Check sheet for the modelled part. Datum: model origin and axes. Units: mm. Face numbers are marked on the shaded views. A direction names the side the tool comes from. Coordinates: 2 decimals unless noted, no trailing zeros. Loops run counter-clockwise (first coordinate to the right, second up) from the corner with the lowest first, then second, coordinate; pieces in that order, holes last. Notation, with made-up numbers: M 26,-38 L 55,-38 A29 cw 55,-3 Z; hole C -13,-21.75 d2. An arc over 180 degrees is marked long. Return JSON: item names as keys, results as strings.
from build123d import *

# Parameters (mm, degrees)
SKETCH2_W                   = 191
SKETCH2_H                   = 130
BOSS_EXTRUDE1_DEPTH         = 35
SKETCH10_W                  = 35
SKETCH10_H                  = 130
BOSS_EXTRUDE2_DEPTH         = 101
TAP_DRILL_FOR_M4_TAP2_D     = 3.3
TAP_DRILL_FOR_M4_TAP2_DEPTH = 6
TAP_DRILL_FOR_M4_TAP2_TIP   = 0.991420021
TAP_DRILL_FOR_M4_TAP3_D     = 3.3
TAP_DRILL_FOR_M4_TAP3_DEPTH = 6
TAP_DRILL_FOR_M4_TAP3_TIP   = 0.991420021
CUT_EXTRUDE1_DEPTH          = 205.770603359
F_8_0MM_DOWEL_HOLE1_D       = 8
CUT_EXTRUDE3_DEPTH          = 30
F_8_0MM_DOWEL_HOLE2_D       = 8
F_8_0MM_DOWEL_HOLE2_DEPTH   = 10
F_8_0MM_DOWEL_HOLE2_TIP     = 2.403442476
F_12_0MM_DOWEL_HOLE1_D      = 12
F_12_0MM_DOWEL_HOLE1_DEPTH  = 10
F_12_0MM_DOWEL_HOLE1_TIP    = 3.605163714


with BuildPart() as part:
    # Sketch2 → Boss-Extrude1 (new body)
    with BuildSketch(Plane(origin=(0, 0, 0), x_dir=(0, 0, -1), z_dir=(1, 0, 0))):
        with Locations((95.5, 0)):
            Rectangle(SKETCH2_W, SKETCH2_H)
    extrude(amount=BOSS_EXTRUDE1_DEPTH)

    # Sketch10 → Boss-Extrude2 (add)
    with BuildSketch(Plane.XY):
        with Locations((17.5, 0)):
            Rectangle(SKETCH10_W, SKETCH10_H)
    extrude(amount=BOSS_EXTRUDE2_DEPTH)

    # Tap Drill for M4 Tap2
    with Locations(Plane(origin=(0, 0, -191), x_dir=(-1, 0, 0), z_dir=(0, 0, -1))):
        with Locations((-40, 35), (-10, 35), (-10, -35), (-40, -35)):
            Hole(TAP_DRILL_FOR_M4_TAP2_D / 2, depth=TAP_DRILL_FOR_M4_TAP2_DEPTH)
            with Locations((0, 0, -(TAP_DRILL_FOR_M4_TAP2_DEPTH + TAP_DRILL_FOR_M4_TAP2_TIP / 2))):  # 118° drill point
                Cone(0, TAP_DRILL_FOR_M4_TAP2_D / 2, TAP_DRILL_FOR_M4_TAP2_TIP, mode=Mode.SUBTRACT)

    # Tap Drill for M4 Tap3
    with Locations(Plane.XY.offset(101)):
        with Locations((10, 35), (40, 35), (40, -35), (10, -35)):
            Hole(TAP_DRILL_FOR_M4_TAP3_D / 2, depth=TAP_DRILL_FOR_M4_TAP3_DEPTH)
            with Locations((0, 0, -(TAP_DRILL_FOR_M4_TAP3_DEPTH + TAP_DRILL_FOR_M4_TAP3_TIP / 2))):  # 118° drill point
                Cone(0, TAP_DRILL_FOR_M4_TAP3_D / 2, TAP_DRILL_FOR_M4_TAP3_TIP, mode=Mode.SUBTRACT)

    # Sketch23 → Cut-Extrude1 (cut, through all)
    with BuildSketch(Plane.ZY):
        with BuildLine():
            Line((-65, 25), (-65, -25))
            ThreePointArc((-65, -25), (-63.535533906, -28.535533906), (-60, -30))
            Line((-60, -30), (0, -30))
            ThreePointArc((0, -30), (3.535533906, -28.535533906), (5, -25))
            Line((5, -25), (5, 25))
            ThreePointArc((5, 25), (3.535533906, 28.535533906), (0, 30))
            Line((0, 30), (-60, 30))
            ThreePointArc((-60, 30), (-63.535533906, 28.535533906), (-65, 25))
        make_face()
    extrude(amount=-CUT_EXTRUDE1_DEPTH, mode=Mode.SUBTRACT)

    # Ø8.0mm Dowel Hole1 (through all)
    with Locations(Plane(origin=(35, 0, 0), x_dir=(0, 0, -1), z_dir=(1, 0, 0))):
        with Locations((-88, 50), (-88, -50), (178, -50), (178, 50)):
            Hole(F_8_0MM_DOWEL_HOLE1_D / 2)

    # Sketch35 → Cut-Extrude3 (cut)
    with BuildSketch(Plane.ZY):
        with BuildLine():
            Line((-151, 55), (-85, 55))
            ThreePointArc((-85, 55), (-77.928932188, 52.071067812), (-75, 45))
            Line((-75, 45), (-75, -45))
            ThreePointArc((-75, -45), (-77.928932188, -52.071067812), (-85, -55))
            Line((-85, -55), (-151, -55))
            ThreePointArc((-151, -55), (-158.071067812, -52.071067812), (-161, -45))
            Line((-161, -45), (-161, 45))
            ThreePointArc((-161, 45), (-158.071067812, 52.071067812), (-151, 55))
        make_face()
        with BuildLine():
            Line((25, 55), (61, 55))
            ThreePointArc((61, 55), (68.071067812, 52.071067812), (71, 45))
            Line((71, 45), (71, -45))
            ThreePointArc((71, -45), (68.071067812, -52.071067812), (61, -55))
            Line((61, -55), (25, -55))
            ThreePointArc((25, -55), (17.928932188, -52.071067812), (15, -45))
            Line((15, -45), (15, 45))
            ThreePointArc((15, 45), (17.928932188, 52.071067812), (25, 55))
        make_face()
    extrude(amount=-CUT_EXTRUDE3_DEPTH, mode=Mode.SUBTRACT)

    # Ø8.0mm Dowel Hole2
    with Locations(Plane(origin=(0, -55, 0), x_dir=(1, 0, 0), z_dir=(0, 1, 0))):
        with Locations((15, 133), (15, 104), (15, -43)):
            Hole(F_8_0MM_DOWEL_HOLE2_D / 2, depth=F_8_0MM_DOWEL_HOLE2_DEPTH)
            with Locations((0, 0, -(F_8_0MM_DOWEL_HOLE2_DEPTH + F_8_0MM_DOWEL_HOLE2_TIP / 2))):  # 118° drill point
                Cone(0, F_8_0MM_DOWEL_HOLE2_D / 2, F_8_0MM_DOWEL_HOLE2_TIP, mode=Mode.SUBTRACT)

    # Ø12.0mm Dowel Hole1
    with Locations(Plane(origin=(0, 65, 0), x_dir=(1, 0, 0), z_dir=(0, 1, 0))):
        with Locations((15, 133), (15, 104), (15, -43)):
            Hole(F_12_0MM_DOWEL_HOLE1_D / 2, depth=F_12_0MM_DOWEL_HOLE1_DEPTH)
            with Locations((0, 0, -(F_12_0MM_DOWEL_HOLE1_DEPTH + F_12_0MM_DOWEL_HOLE1_TIP / 2))):  # 118° drill point
                Cone(0, F_12_0MM_DOWEL_HOLE1_D / 2, F_12_0MM_DOWEL_HOLE1_TIP, mode=Mode.SUBTRACT)


solid = part.part
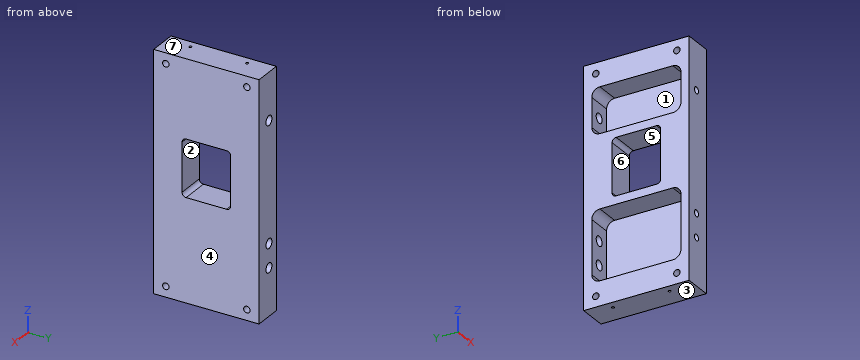
1) Draft check along Z on the marked faces 4, 5, 6 and 7. Enter one of: +Z half, -Z half, draft (parallel to the pull), parting line (faces both ways), or undercut.
Answers:
{"face 4": "draft", "face 5": "undercut", "face 6": "undercut", "face 7": "+Z half"}
2) Section check A-A on z = -178. Record the cut outline in (x, y), then the cut area to 3 significant figures.
Answers:
{"outline": "M 0,-65 L 35,-65 L 35,-54 L 0,-54 Z; M 0,-46 L 35,-46 L 35,46 L 0,46 Z; M 0,54 L 35,54 L 35,65 L 0,65 Z", "area": "3,990 mm²"}
3) Scan lines: line 1 along Z through (x, y) = (24, -23.5); line 2 along Z through (x, y) = (15, 59.5); line 3 along Y through (x, z) = (7, 88). Record each from-to range of solid material in increasing order. Write a range as [from, to].
Answers:
{"line 1": "[-191, -161], [-75, -65], [5, 15], [71, 101]", "line 2": "[-191, -139], [-127, -110], [-98, 37], [49, 101]", "line 3": "[-65, -54], [-46, 46], [54, 65]"}
4) Set-up check for the marked faces 1, 2 and 3: record each of +Z, -Z, +X, -X, +Y, -Y from which the full face is reachable in a straight line by a thin tool's end or side.
Answers:
{"face 1": "-X", "face 2": "+X, -X", "face 3": "-Z, +X, -X, +Y, -Y"}
5) Section check C-C on x = 4.5. Count the separate pieces of the cut face and the enclosed holes in it, then the cut area to 3 significant figures.
Answers:
{"separate pieces": "1", "enclosed holes": "7", "area": "18,100 mm²"}
6) Go/stop test with flat-tipped pins: pin 1 Ø7 at (x, z) = (15, -104) entering from -Y; pin 2 Ø5.5 at (x, y) = (10, 35) entering from -Z; pin 3 Ø5 at (y, z) = (36.5, -112) entering from -X; pin 4 Ø11 at (x, z) = (15, 43) entering from +Y. Record where each tip stops, or that it passes through.
Answers:
{"pin 1": "through", "pin 2": "z = -191", "pin 3": "x = 30", "pin 4": "y = -55"}
7) Section check B-B on y = -17. Record the cut outline in (x, z), then the cut area to 3 significant figures.
Answers:
{"outline": "M 0,-191 L 35,-191 L 35,-65 L 0,-65 L 0,-75 L 30,-75 L 30,-161 L 0,-161 Z; M 0,5 L 35,5 L 35,101 L 0,101 L 0,71 L 30,71 L 30,15 L 0,15 Z", "area": "3,510 mm²"}
8) Section check D-D on z = -104. Record the cut outline in (x, y), then the cut area to 3 significant figures.
Answers:
{"outline": "M 0,-65 L 11,-65 L 11,-55 L 0,-55 Z; M 0,55 L 9,55 L 9,65 L 0,65 Z; M 19,-65 L 35,-65 L 35,65 L 21,65 L 21,55 L 30,55 L 30,-55 L 19,-55 Z", "area": "1,050 mm²"}
